Read the model definition and answer for the solid it produces. Units are mm, in the model's axes. Face numbers are marked on the shaded views. A direction names the side the tool comes from. Round coordinates to 2 decimals unless told otherwise and drop trailing zeros. Write each loop counter-clockwise with the first axis right and the second up, starting at its lowest first coordinate (ties: lowest second). Pieces come first, ordered by that corner, then holes. Notation, with made-up numbers: (23.25, 55) - (82.25, 55) arc R19 cw to (82.25, 88) - close; hole circle Ø1 at (-19.5, 27). An arc over 180 degrees is marked (long way). Use one line per item in the form item = value. Start each with the question number.
1) Consider line 1 along X through (y, z) = (10.16, 1.1); line 2 along Z through (x, y) = (20.32, 3.5); line 3 along Y through (x, z) = (7.62, 0.8). Determine where each line is inside the solid, lowest interval first. Write a range as from..to.
2) The part is cut by section A-A, the plane x = 20.32. Give the vertices of the cut face in (y, z) (3 decimals).
3) The part is cut by section D-D, the plane x = 7.62. Give the vertices of the cut face in (y, z) (3 decimals), plus the area to 3 significant figures.
4) This flat-tipped pin is pushed along its axis until it touches: pin 1 (5.5 mm diameter, centred on x = 32.5, y = 11.5, fed in from +Z) (3 decimals). Where does it stop, or does it pass through?
5) The part is cut by section C-C, the plane y = 18.5. Give the vertices of the cut face in (x, z), plus the area to 3 significant figures.
6) For a pull along X with two mould halves and no side action, classify the marked faces 3, 4 and 5 as released by +X, released by -X, zero draft, split by the parting line, or undercut.
7) For the marked faces 1 and 2, determine the directions among +Z, -Z, +X, -X, +Y, -Y from which every point of the face is accessible in a straight line to the end or side of a thin tool.
8) The part is cut by section B-B, the plane z = 7. Give the vertices of the cut face in (x, y).
from build123d import *

# Parameters (mm, degrees)
SKETCH1_W                                     = 40.64
SKETCH1_H                                     = 20.32
BOSS_EXTRUDE2_DEPTH                           = 12.7
CBORE_FOR_1_4_SOCKET_HEAD_CAP_SCREW1_AT_COUNT = 2
CBORE_FOR_1_4_SOCKET_HEAD_CAP_SCREW1_AT_PITCH = 25.4
HOLE1_D                                       = 10.2616
HOLE1_DEPTH                                   = 9.525
F_4_40_TAPPED_HOLE1_D                         = 2.2606


with BuildPart() as part:
    # Sketch1 → Boss-Extrude2 (new body)
    with BuildSketch(Plane.XY):
        with Locations((20.32, 10.16)):
            Rectangle(SKETCH1_W, SKETCH1_H)
    extrude(amount=BOSS_EXTRUDE2_DEPTH)

    # Sketch3 → CBORE for 1/4 Socket Head Cap Screw1 (revolve, cut)
    with BuildSketch(Plane(origin=(7.62, 10.16, 12.7), x_dir=(0, -1, 0), z_dir=(1, 0, 0))):
        Polygon((0, 0), (0, 12.7), (3.3782, 12.7), (3.3782, 9.525), (5.55625, 9.525), (5.55625, 0.2159), (5.77215, 0), align=None)
    cbore_for_1_4_socket_head_cap_screw1 = revolve(axis=Axis((7.62, 10.16, 19.05), (0, 0, -1)), mode=Mode.SUBTRACT)

    # CBORE for 1/4 Socket Head Cap Screw1 at: CBORE for 1/4 Socket Head Cap Screw1 ×2
    with Locations(*[(i * CBORE_FOR_1_4_SOCKET_HEAD_CAP_SCREW1_AT_PITCH, 0, 0) for i in range(1, CBORE_FOR_1_4_SOCKET_HEAD_CAP_SCREW1_AT_COUNT)]):
        add(cbore_for_1_4_socket_head_cap_screw1, mode=Mode.SUBTRACT)

    # Hole1
    with Locations(Plane.XY.offset(12.7)):
        with Locations((20.32, 10.16)):
            Hole(HOLE1_D / 2, depth=HOLE1_DEPTH)

    # #4-40 Tapped Hole1 (through all)
    with Locations(Plane(origin=(0, 20.32, 0), x_dir=(1, 0, 0), z_dir=(0, 1, 0))):
        with Locations((20.32, -10.16), (20.32, -6.35)):
            Hole(F_4_40_TAPPED_HOLE1_D / 2)


solid = part.part
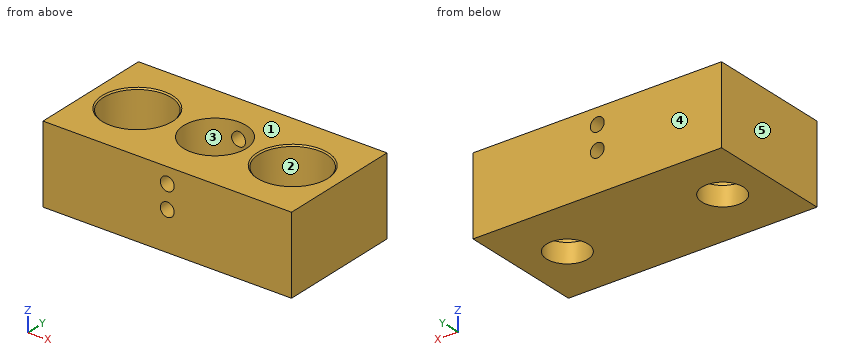
Geometry results:
q1.line_1 = 0..4.24, 11..29.64, 36.4..40.64
q1.line_2 = 0..5.22, 7.48..9.03, 11.29..12.7
q1.line_3 = 0..6.78, 13.54..20.32
q2.outline = (0, 0) - (20.32, 0) - (20.32, 5.22) - (15.291, 5.22) - (15.291, 3.175) - (5.029, 3.175) - (5.029, 5.22) - (0, 5.22) - close; (0, 7.48) - (5.029, 7.48) - (5.029, 9.03) - (0, 9.03) - close; (0, 11.29) - (5.029, 11.29) - (5.029, 12.7) - (0, 12.7) - close; (15.291, 7.48) - (20.32, 7.48) - (20.32, 9.03) - (15.291, 9.03) - close; (15.291, 11.29) - (20.32, 11.29) - (20.32, 12.7) - (15.291, 12.7) - close
q3.outline = (0, 0) - (6.782, 0) - (6.782, 3.175) - (4.604, 3.175) - (4.604, 12.484) - (4.388, 12.7) - (0, 12.7) - close; (13.538, 0) - (20.32, 0) - (20.32, 12.7) - (15.932, 12.7) - (15.716, 12.484) - (15.716, 3.175) - (13.538, 3.175) - close
q3.area = 131 mm2
q4.pin_1 = 3.175
q5.outline = (0, 0) - (40.64, 0) - (40.64, 12.7) - (0, 12.7) - close; hole circle Ø2.26 at (20.32, 6.35); hole circle Ø2.26 at (20.32, 10.16)
q5.area = 508 mm2
q6.face_3 = undercut
q6.face_4 = zero draft
q6.face_5 = released by -X
q7.face_1 = +Z, +X, -X, +Y, -Y
q7.face_2 = +Z
q8.outline = (0, 0) - (19.4, 0) - (19.4, 5.11) arc R5.13 cw to (19.4, 15.21) - (19.4, 20.32) - (0, 20.32) - close; (21.24, 0) - (40.64, 0) - (40.64, 20.32) - (21.24, 20.32) - (21.24, 15.21) arc R5.13 cw to (21.24, 5.11) - close; hole circle Ø11.11 at (7.62, 10.16); hole circle Ø11.11 at (33.02, 10.16)
